Design review of the part built by this model. Coordinates are the model's own, in mm. A direction names the side the tool comes from. Round coordinates to 2 decimals unless told otherwise and drop trailing zeros. Loops run counter-clockwise (first coordinate to the right, second up) from the corner with the lowest first, then second, coordinate; pieces in that order, holes last. Notation, with made-up numbers: M 62.25,-38.75 L 99.25,-38.75 A17 ccw 99.25,-32.75 Z; hole C -27,65 d1. An arc over 180 degrees is marked long. One line per item, written item: value. Start each with the question number.
Item 1: We need section D-D (y = -9.5). Write out the cut boundary in (x, z).
Item 2: Clearance check with flat-ended pins moving along their axes: pin 1 (4 mm diameter, centred on x = -9, y = -4.5, fed in from -Z); pin 2 (5 mm diameter, centred on y = 5.5, z = -6, fed in from -X); pin 3 (4 mm diameter, centred on x = 0, y = 9.5, fed in from +Z); pin 4 (9 mm diameter, centred on x = 0, y = 9.5, fed in from -Z). State where each tip first meets the part, or that it passes through.
Item 3: Mouldability with a two-part tool opening along X and no side actions: class faces 1 (the flat face through (0, 6, -8)), 2 (the cylindrical face through (5.96, -1.88, -3.94)), 3 (the cylindrical face through (0, 6, 5)) as released by +X, released by -X, zero draft, split by the parting line, or undercut.
Item 4: For line 1 along Y through (x, z) = (0, 2.2); line 2 along Y through (x, z) = (0, 5.7); line 3 along X through (y, z) = (0, -0.5), list the stretches that pass through material, from the lowest coordinate up.
Item 5: For faces 4 (the cylindrical face through (0, -6, 5)), 5 (the flat face through (3, 6, 0)), 6 (the cylindrical face through (6.75, 0.05, 3.55)), list the 3-axis set-ups (+Z, -Z, +X, -X, +Y, -Y) from which the entire face can be reached by the end or side of a thin tool; tool diameter is ignored.
Item 6: We need section C-C (z = -2.75). Write out the cut boundary in (x, y).
Item 7: We need section B-B (x = 8). Write out the cut boundary in (y, z), then the cut area to 3 significant figures.
Item 8: We need section A-A (y = 0). Write out the cut boundary in (x, z), then the cut area to 3 significant figures.
from build123d import *

# Parameters (mm, degrees)
F0_R          = 12.5
F1_DEPTH      = 7
F2_R          = 1.5
F3_DEPTH      = 7.001
F4_R          = 3.5
F5_DEPTH      = 4
F6_R          = 6.25
F6_R_2        = 5
F7_DEPTH      = 8
F8_R          = 5.5
F9_DEPTH      = 7.001
F9_DEPTH_BACK = 8.001
F10_R         = 1.25
F11_DEPTH     = 15.001


with BuildPart() as f1:
    # F0 (on Top) → F1 (new body)
    with BuildSketch(Plane.XY):
        Circle(F0_R)
    extrude(amount=F1_DEPTH)

    # F2 (on face) → F3 (cut, through all)
    with BuildSketch(Plane.XY.offset(7)):
        with Locations((0, 9.5)):
            Circle(F2_R)
        with Locations((0, -9.5)):
            Circle(F2_R)
    extrude(amount=-F3_DEPTH, mode=Mode.SUBTRACT)

    # F4 (on face) → F5 (cut, through all)
    with BuildSketch(Plane.XY.offset(7)):
        with Locations((0, 9.5)):
            Circle(F4_R)
        with Locations((0, -9.5)):
            Circle(F4_R)
    extrude(amount=-F5_DEPTH, mode=Mode.SUBTRACT)

    # F6 (on face) → F7 (join)
    with BuildSketch(Plane(origin=(0, 0, 0), x_dir=(1, 0, 0), z_dir=(0, 0, -1))):
        Circle(F6_R)
        Circle(F6_R_2, mode=Mode.SUBTRACT)
    extrude(amount=F7_DEPTH)

    # F8 (on face) → F9 (cut, two sides)
    with BuildSketch(Plane(origin=(0, 0, 0), x_dir=(1, 0, 0), z_dir=(0, 0, -1))) as f9_sk:
        Circle(F8_R)
    extrude(amount=-F9_DEPTH, mode=Mode.SUBTRACT)
    extrude(f9_sk.sketch, amount=F9_DEPTH_BACK, mode=Mode.SUBTRACT)

    # F10 (on face) → F11 (cut, through all)
    with BuildSketch(Plane.XY.offset(7)):
        with Locations((8, 0)):
            Circle(F10_R)
        with Locations((-8, 0)):
            Circle(F10_R)
    extrude(amount=-F11_DEPTH, mode=Mode.SUBTRACT)


solid = f1.part
A:
1. outline: M -8.12,0 L -1.5,0 L -1.5,3 L -3.5,3 L -3.5,7 L -8.12,7 Z; M 1.5,0 L 8.12,0 L 8.12,7 L 3.5,7 L 3.5,3 L 1.5,3 Z
2. pin 1: z = 0
2. pin 2: x = -5.48
2. pin 3: z = 3
2. pin 4: z = -8
3. face 1: zero draft
3. face 2: split by the parting line
3. face 3: undercut
4. line 1: -12.5 to -11, -8 to -5.5, 5.5 to 8, 11 to 12.5
4. line 2: -6 to -5.5, 5.5 to 6
4. line 3: -6.25 to -5.5, 5.5 to 6.25
5. face 4: +Z
5. face 5: -Z
5. face 6: +Z, -Z
6. outline: C 0,0 d12.5; hole C 0,0 d11
7. outline: M -9.6,0 L -1.25,0 L -1.25,7 L -9.6,7 Z; M 1.25,0 L 9.6,0 L 9.6,7 L 1.25,7 Z
7. area: 117 mm2
8. outline: M -12.5,0 L -9.25,0 L -9.25,7 L -12.5,7 Z; M -6.75,0 L -6.25,0 L -6.25,-8 L -5.5,-8 L -5.5,7 L -6.75,7 Z; M 5.5,-8 L 6.25,-8 L 6.25,0 L 6.75,0 L 6.75,7 L 5.5,7 Z; M 9.25,0 L 12.5,0 L 12.5,7 L 9.25,7 Z
8. area: 75.0 mm2
